Verification items for the finished model (mm, model axes). A direction names the side the tool comes from. Round coordinates to 2 decimals unless told otherwise and drop trailing zeros. Loops run counter-clockwise (first coordinate to the right, second up) from the corner with the lowest first, then second, coordinate; pieces in that order, holes last. Notation, with made-up numbers: (39.25, 3.25) - (47.25, 3.25) arc R10 ccw to (47.25, 17.25) - close; hole circle Ø8 at (78.25, 59.25). An arc over 180 degrees is marked (long way). Use a Markdown table: item, result. Add a question column.
```python
from build123d import *

# Parameters (mm, degrees)
SKETCH1_W           = 71.7
SKETCH1_H           = 101.4
BOSS_EXTRUDE1_DEPTH = 11.1
CUT_EXTRUDE1_DEPTH  = 62.3
SKETCH6_W           = 87
SKETCH6_H           = 3.1
CUT_EXTRUDE2_DEPTH  = 2.2
FILLET1_R           = 0.5
FILLET2_R           = 1
SKETCH7_R           = 1.5
CUT_EXTRUDE3_DEPTH  = 4
SKETCH8_R           = 1.5
CUT_EXTRUDE4_DEPTH  = 4


with BuildPart() as part:
    # Sketch1 → Boss-Extrude1 (new body)
    with BuildSketch(Plane(origin=(0, 0, 0), x_dir=(1, 0, 0), z_dir=(0, 1, 0))):
        Rectangle(SKETCH1_W, SKETCH1_H)
    extrude(amount=BOSS_EXTRUDE1_DEPTH)

    # Sketch5 → Cut-Extrude1 (cut)
    with BuildSketch(Plane(origin=(35.85, 0, 0), x_dir=(0, 0, -1), z_dir=(1, 0, 0))):
        Polygon((-41.3, 18.36393321), (-41.3, 7.1), (-43.5, 7.1), (-43.5, 4), (43.5, 4), (43.5, 7.1), (41.3, 7.1), (41.3, 18.36393321), align=None)
    extrude(amount=-CUT_EXTRUDE1_DEPTH, mode=Mode.SUBTRACT)

    # Sketch6 → Cut-Extrude2 (cut)
    with BuildSketch(Plane(origin=(-26.45, 0, 0), x_dir=(0, 0, -1), z_dir=(1, 0, 0))):
        with Locations((0, 5.55)):
            Rectangle(SKETCH6_W, SKETCH6_H)
    extrude(amount=-CUT_EXTRUDE2_DEPTH, mode=Mode.SUBTRACT)

    # Fillet1
    fillet1_edges = [part.edges().sort_by_distance(p)[0] for p in [
        (-26.45, 9.1, -41.3),
        (4.7, 7.1, -41.3),
        (3.6, 7.1, -43.5),
        (3.6, 4, -43.5),
        (3.6, 4, 43.5),
        (3.6, 7.1, 43.5),
        (-26.45, 9.1, 41.3),
        (4.7, 7.1, 41.3),
        (-26.45, 7.1, 0),
        (-28.65, 7.1, 0),
        (-28.65, 5.55, -43.5),
        (-28.65, 4, 0),
        (-28.65, 5.55, 43.5),
    ]]
    fillet(fillet1_edges, radius=FILLET1_R)

    # Fillet2
    fillet2_edges = [part.edges().sort_by_distance(p)[0] for p in [
        (0, 11.1, -50.7),
        (-35.85, 11.1, 0),
        (0, 11.1, 50.7),
        (-35.85, 5.55, -50.7),
        (-35.85, 5.55, 50.7),
    ]]
    fillet(fillet2_edges, radius=FILLET2_R)

    # Sketch7 → Cut-Extrude3 (cut)
    with BuildSketch(Plane(origin=(0, 11.1, 0), x_dir=(1, 0, 0), z_dir=(0, 1, 0))):
        with Locations(Location((-31.75, -6.65790951, 0), (0, 0, 270))):
            Circle(SKETCH7_R)
        with Locations(Location((-31.75, 6.65790951, 0), (0, 0, 90))):
            Circle(SKETCH7_R)
    extrude(amount=-CUT_EXTRUDE3_DEPTH, mode=Mode.SUBTRACT)

    # Sketch8 → Cut-Extrude4 (cut)
    with BuildSketch(Plane(origin=(0, 11.1, 0), x_dir=(1, 0, 0), z_dir=(0, 1, 0))):
        with Locations(Location((29.19209049, -46.6, 0), (0, 0, 270))):
            Circle(SKETCH8_R)
        with Locations(Location((29.19209049, 46.6, 0), (0, 0, 270))):
            Circle(SKETCH8_R)
    extrude(amount=-CUT_EXTRUDE4_DEPTH, mode=Mode.SUBTRACT)


solid = part.part
```
Q1. Section check A-A on x = -31.75. Record the cut outline in (y, z), plus the area to 3 significant figures.
Q2. Set-up check for faces 1 (the face through (-28, 11.1, 0)), 2 (the face through (-28.65, 6, 1)), 3 (the face through (-30.485, 9.128, 7.464)), 4 (the face through (-1, 0, -1)), 5 (the face through (5, 9, 41.3)): record each of +Z, -Z, +X, -X, +Y, -Y from which the full face is reachable in a straight line by a thin tool's end or side.
Q3. Release check for a two-part mould opening along Z. For faces 6 (the face through (28.618, 9.128, -45.214)), 7 (the face through (0, 5, -50.7)), 8 (the face through (-35.85, 5, 1)), 9 (the face through (-31.175, 9.128, -8.044)) record: +Z half, -Z half, draft (parallel to the pull), parting line (faces both ways), or undercut.
Q4. Go/stop test with flat-tipped pins: pin 1 Ø2.5 at (x, z) = (-31.75, 6.66) entering from +Y; pin 2 Ø19 at (x, z) = (-7.5, 9) entering from +Y; pin 3 Ø1 at (y, z) = (5, -19) entering from +X. Record where each tip stops, or that it passes through.
Q5. Section check B-B on z = -46.6. Record the cut outline in (x, y), plus the area to 3 significant figures.
Q6. Section check D-D on z = -20. Record the cut outline in (x, y), plus the area to 3 significant figures.
Q7. Thickness scan on line 1 along Z through (x, y) = (-13, 8.75); line 2 along Y through (x, z) = (-18.5, 42.5); line 3 along Y through (x, z) = (13, 4). Record the ranges inside material, lowest first.
Q8. Section check C-C on x = -18. Record the cut outline in (y, z), plus the area to 3 significant figures.
Determined:
| question | item | result |
|---|---|---|
| 1 | outline | (0, -50.7) - (10.1, -50.7) arc R1 ccw to (11.1, -49.7) - (11.1, -8.16) - (7.1, -8.16) - (7.1, -5.16) - (11.1, -5.16) - (11.1, 5.16) - (7.1, 5.16) - (7.1, 8.16) - (11.1, 8.16) - (11.1, 49.7) arc R1 ccw to (10.1, 50.7) - (0, 50.7) - close |
| 1 | area | 1,100 mm² |
| 2 | face 1 | +Z, -Z, +X, -X, +Y |
| 2 | face 2 | +X |
| 2 | face 3 | +Y |
| 2 | face 4 | +Z, -Z, +X, -X, -Y |
| 2 | face 5 | +X, +Y |
| 3 | face 6 | undercut |
| 3 | face 7 | -Z half |
| 3 | face 8 | draft |
| 3 | face 9 | undercut |
| 4 | pin 1 | stops at y = 7.1 |
| 4 | pin 2 | stops at y = 4 |
| 4 | pin 3 | stops at x = -28.65 |
| 5 | outline | (-35.85, 0) - (35.85, 0) - (35.85, 11.1) - (30.69, 11.1) - (30.69, 7.1) - (27.69, 7.1) - (27.69, 11.1) - (-34.85, 11.1) arc R1 ccw to (-35.85, 10.1) - close |
| 5 | area | 784 mm² |
| 6 | outline | (-35.85, 0) - (35.85, 0) - (35.85, 4) - (-28.15, 4) arc R0.5 cw to (-28.65, 4.5) - (-28.65, 6.6) arc R0.5 cw to (-28.15, 7.1) - (-26.95, 7.1) arc R0.5 ccw to (-26.45, 7.6) - (-26.45, 11.1) - (-34.85, 11.1) arc R1 ccw to (-35.85, 10.1) - close |
| 6 | area | 347 mm² |
| 7 | line 1 | z = -50.7 to -41.3, 41.3 to 50.7 |
| 7 | line 2 | y = 0 to 4, 7.1 to 11.1 |
| 7 | line 3 | y = 0 to 4 |
| 8 | outline | (0, -50.7) - (10.1, -50.7) arc R1 ccw to (11.1, -49.7) - (11.1, -41.3) - (7.6, -41.3) arc R0.5 ccw to (7.1, -41.8) - (7.1, -43) arc R0.5 cw to (6.6, -43.5) - (4.5, -43.5) arc R0.5 cw to (4, -43) - (4, 43) arc R0.5 cw to (4.5, 43.5) - (6.6, 43.5) arc R0.5 cw to (7.1, 43) - (7.1, 41.8) arc R0.5 ccw to (7.6, 41.3) - (11.1, 41.3) - (11.1, 49.7) arc R1 ccw to (10.1, 50.7) - (0, 50.7) - close |
| 8 | area | 525 mm² |
